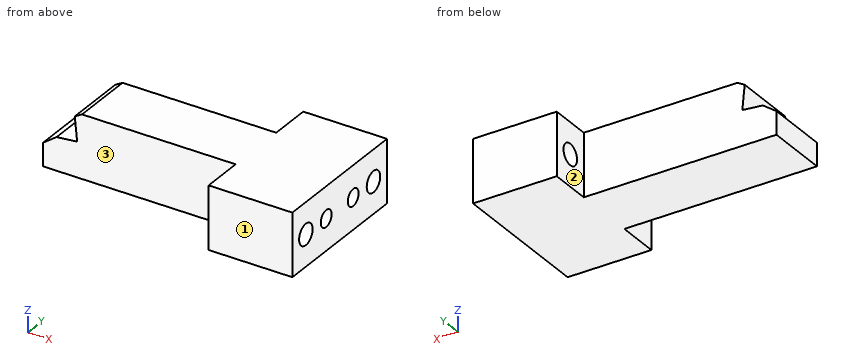
from build123d import *

# Parameters (mm, degrees)
F0_W      = 20
F0_H      = 7.5
F1_DEPTH  = 35
F2_W      = 36.682897
F2_H      = 10
F3_DEPTH  = 15.001
F4_R      = 2.5
F5_DEPTH  = 20.001
F7_W      = 23.5301591456
F7_H      = 12.1317058802
F8_DEPTH  = 25
F6_R      = 2
F11_DEPTH = 6


with BuildPart() as f1:
    # F0 (on Front) → F1 (new body)
    with BuildSketch(Plane.XZ):
        Polygon((61.530317, -30.704832), (61.530317, -23.204832), (24.84742, -23.204832), (23.115369, -24.204832), (23.679145, -29.89786), (18.780462, -30.382973), (15.530317, -32.714615), (15.530317, -38.204832), (61.530317, -38.204832), align=None)
        with Locations((71.530317, -26.954832)):
            Rectangle(F0_W, F0_H)
        with Locations((71.530317, -34.454832)):
            Rectangle(F0_W, F0_H)
    extrude(amount=F1_DEPTH)

    # F2 (on face) → F3 (cut, through all)
    with BuildSketch(Plane.XY.offset(-23.204832)):
        with Locations((43.1888685, -5)):
            Rectangle(F2_W, F2_H)
        Polygon((24.84742, -10), (24.84742, 0), (23.679145, 0), (23.115369, 0), (18.780462, 0), (15.530317, 0), (15.530317, -10), (18.780462, -10), (23.115369, -10), (23.679145, -10), align=None)
        with Locations((43.1888685, -30)):
            Rectangle(F2_W, F2_H)
        Polygon((24.84742, -35), (24.84742, -25), (23.679145, -25), (23.115369, -25), (18.780462, -25), (15.530317, -25), (15.530317, -35), (18.780462, -35), (23.115369, -35), (23.679145, -35), align=None)
    extrude(amount=-F3_DEPTH, mode=Mode.SUBTRACT)

    # F4 (on face) → F5 (cut, through all)
    with BuildSketch(Plane(origin=(61.530317, 0, 0), x_dir=(0, -1, 0), z_dir=(-1, 0, 0))):
        with Locations((30, -30.704832)):
            Circle(F4_R)
        with Locations((5, -30.704832)):
            Circle(F4_R)
    extrude(amount=-F5_DEPTH, mode=Mode.SUBTRACT)

    # F6 (on face) → F11 (cut)
    with BuildSketch(Plane.YZ.offset(81.530317)):
        with Locations((-12.5, -30.704832)):
            Circle(F6_R)
        with Locations((-22.5, -30.704832)):
            Circle(F6_R)
    extrude(amount=-F11_DEPTH, mode=Mode.SUBTRACT)


with BuildPart() as f8:
    # F7 (on Right) → F8 (new body)
    with BuildSketch(Plane.YZ):
        with Locations((-54.0060605854, 53.4663982689)):
            Rectangle(F7_W, F7_H)
    extrude(amount=F8_DEPTH)


with BuildPart() as f9_1:
    # F9: copy of F8
    add(f8.part.moved(Location((0, -65, 0))))


solid = f1.part
CAD build for the part. Positions are in the model's coordinates, mm. Face numbers are marked on the shaded views. A direction names the side the tool comes from. Give positions to 0.01 mm unless a question says otherwise; leave off trailing zeros. Order: outer loops, then holes, each group sorted by start corner. A loop starts at its lowest first (then second) coordinate and runs counter-clockwise, first axis right, second up. Notation, with made-up numbers: (77.25, 30.5) -> (109.25, 30.5) arc R9 ccw to (109.25, 39.5) -> close; hole circle Ø6 at (40.5, -9.75). An arc over 180 degrees is marked (long way). Return JSON: item names as keys, results as strings.
Q1. Drill centre lines: line 1 (Z direction, x = 68.5, y = -30); line 2 (Y direction, x = 78, z = -32); line 3 (Y direction, x = 63.5, z = -29). Where is each one in solid material? Low to high.
Working result:
{"line 1": "-38.2 to -33.2, -28.2 to -23.2", "line 2": "-35 to -32.14, -27.86 to -24.02, -20.98 to -14.02, -10.98 to -7.14, -2.86 to 0", "line 3": "-35 to -31.83, -28.17 to -6.83, -3.17 to 0"}
Q2. Saw through at A-A (y = -30). Write the cut outline in (x, z), then the cut area to 3 significant figures.
Working result:
{"outline": "(61.53, -38.2) -> (81.53, -38.2) -> (81.53, -33.2) -> (61.53, -33.2) -> close; (61.53, -28.2) -> (81.53, -28.2) -> (81.53, -23.2) -> (61.53, -23.2) -> close", "area": "200 mm²"}
Q3. Saw through at B-B (y = -12.5). Write the cut outline in (x, z).
Working result:
{"outline": "(15.53, -38.2) -> (81.53, -38.2) -> (81.53, -32.7) -> (75.53, -32.7) -> (75.53, -28.7) -> (81.53, -28.7) -> (81.53, -23.2) -> (24.85, -23.2) -> (23.12, -24.2) -> (23.68, -29.9) -> (18.78, -30.38) -> (15.53, -32.71) -> close"}
Q4. Saw through at C-C (z = -25.5). Write the cut outline in (x, y).
Working result:
{"outline": "(23.24, -25) -> (61.53, -25) -> (61.53, -35) -> (81.53, -35) -> (81.53, 0) -> (61.53, 0) -> (61.53, -10) -> (23.24, -10) -> close"}
Q5. Flat gauge pins, fed straight in: pin 1 (5 mm diameter, centred on y = -31, z = -28, fed in from -X); pin 2 (1.2 mm diameter, centred on y = -12.5, z = -31.5, fed in from +X); pin 3 (1 mm diameter, centred on x = 37.5, z = -35.5, fed in from -Y). Where does each tip first touch, or does it go through?
Working result:
{"pin 1": "x = 61.53", "pin 2": "x = 75.53", "pin 3": "y = -25"}
Q6. Which spindle directions (+Z, -Z, +X, -X, +Y, -Y) get a long thin tool onto all of the face, cutting with end or side? Do the marked faces 1, 2 and 3. Say none if no direction does.
Working result:
{"face 1": "+Z, -Z, +X, -X, -Y", "face 2": "+Z, -Z, -X, +Y", "face 3": "+Z, -Z, -X, -Y"}
Q7. Saw through at D-D (y = -6.5). Write the cut outline in (x, z), then the cut area to 3 significant figures.
Working result:
{"outline": "(61.53, -38.2) -> (81.53, -38.2) -> (81.53, -32.7) -> (61.53, -32.7) -> close; (61.53, -28.7) -> (81.53, -28.7) -> (81.53, -23.2) -> (61.53, -23.2) -> close", "area": "220 mm²"}
